Design review of the part built by this model. Coordinates are the model's own, in mm. A direction names the side the tool comes from. Give positions to 0.01 mm unless a question says otherwise; leave off trailing zeros. Write each loop counter-clockwise with the first axis right and the second up, starting at its lowest first coordinate (ties: lowest second). Pieces come first, ordered by that corner, then holes. Notation, with made-up numbers: M 50.5,56.25 L 62.5,56.25 A20 ccw 62.5,77.25 Z; hole C 69.5,25 d8. An arc over 180 degrees is marked long. Write each question's results on one line, items separated by ' | '. Start each with the question number.
from build123d import *

# Parameters (mm, degrees)
SKETCH1_R           = 3.175
BOSS_EXTRUDE1_DEPTH = 50.8
SKETCH3_R           = 6.35
BOSS_EXTRUDE2_DEPTH = 2.54


with BuildPart() as part:
    # Sketch1 → Boss-Extrude1 (new body)
    with BuildSketch(Plane.XY):
        Circle(SKETCH1_R)
    extrude(amount=BOSS_EXTRUDE1_DEPTH)

    # Sketch3 → Boss-Extrude2 (add)
    with BuildSketch(Plane.XY.offset(50.8)):
        Circle(SKETCH3_R)
    boss_extrude2 = extrude(amount=BOSS_EXTRUDE2_DEPTH)

    # Mirror1: Boss-Extrude2 across plane
    add(boss_extrude2.mirror(Plane.XY.offset(25.4)))


solid = part.part
Q1. The part is to be moulded in two halves that separate along Z. For faces 3 (the flat face through (0, 0, -2.54)), 4 (the cylindrical face through (-1.38, -6.2, -1.25)), 5 (the flat face through (-2, 3, 50.8)), say which applies: pulls with the +Z half, pulls with the -Z half, needs draft (parallel to the pull), parting line crosses it, or undercut.
Q2. For pin 1 Ø5 at (x, z) = (2, 30) entering from -Y (3 decimals); pin 2 Ø1.5 at (y, z) = (1, 19.5) entering from +X; pin 3 Ø4 at (y, z) = (-2, 3) entering from -X (3 decimals), all flat-tipped, find the tip position at first contact; note any pin that passes through.
Q3. We need section D-D on y = 1.75. Write out the cut boundary in (x, z), and give its area (3 significant figures).
Q4. For faces 1 (the cylindrical face through (-1.38, -6.2, 52.05)), 2 (the flat face through (-2, 3, 0)), list the 3-axis set-ups (+Z, -Z, +X, -X, +Y, -Y) from which the entire face can be reached by the end or side of a thin tool; tool diameter is ignored.
Q5. We need section A-A on y = -3.75. Write out the cut boundary in (x, z).
Q6. We need section B-B on x = -5.25. Write out the cut boundary in (y, z), and give its area (3 significant figures).
Q7. Wall thickness on line 1 along Z through (x, y) = (-3.75, 3.25); line 2 along X through (y, z) = (0.25, 18); line 3 along X through (y, z) = (2.5, 6): over which ranges is each line inside the solid? List them lowest first. Write a range as from..to.
Q8. We need section C-C on x = 0. Write out the cut boundary in (y, z) (3 decimals).
Answer sheet:
1) face 3: pulls with the -Z half | face 4: needs draft | face 5: undercut
2) pin 1: y = -3.175 | pin 2: x = 3.17 | pin 3: x = -3.175
3) outline: M -6.1,-2.54 L 6.1,-2.54 L 6.1,0 L 2.65,0 L 2.65,50.8 L 6.1,50.8 L 6.1,53.34 L -6.1,53.34 L -6.1,50.8 L -2.65,50.8 L -2.65,0 L -6.1,0 Z | area: 331 mm^2
4) face 1: +Z, -Z | face 2: none
5) outline: M -5.12,-2.54 L 5.12,-2.54 L 5.12,0 L -5.12,0 Z; M -5.12,50.8 L 5.12,50.8 L 5.12,53.34 L -5.12,53.34 Z
6) outline: M -3.57,-2.54 L 3.57,-2.54 L 3.57,0 L -3.57,0 Z; M -3.57,50.8 L 3.57,50.8 L 3.57,53.34 L -3.57,53.34 Z | area: 36.3 mm^2
7) line 1: -2.54..0, 50.8..53.34 | line 2: -3.17..3.17 | line 3: -1.96..1.96
8) outline: M -6.35,-2.54 L 6.35,-2.54 L 6.35,0 L 3.175,0 L 3.175,50.8 L 6.35,50.8 L 6.35,53.34 L -6.35,53.34 L -6.35,50.8 L -3.175,50.8 L -3.175,0 L -6.35,0 Z
